Geometry: see drawing. Coordinates: mm, zero at the bounding-box minimum. Coordinates: 2 decimals unless noted, no trailing zeros. Loops run counter-clockwise (first coordinate to the right, second up) from the corner with the lowest first, then second, coordinate; pieces in that order, holes last. Notation, with made-up numbers: (20.5, 85.25) - (41.5, 85.25) arc R30 cw to (41.5, 123.25) - close; hole circle Ø8 at (19.5, -39.5). An arc over 180 degrees is marked (long way). Write item = value, one per line. Start each with the question number.
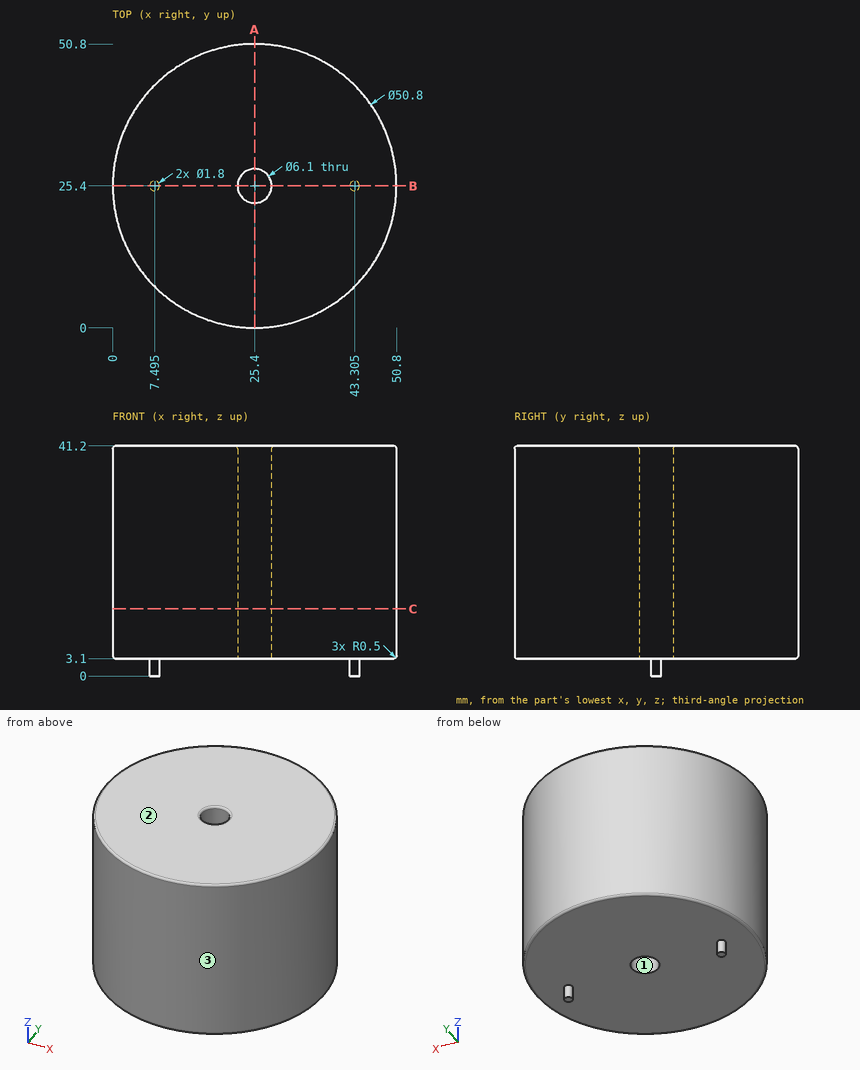
Item 1: Draft query along Y for the marked faces 1, 2 and 3. Return one class per face: released by +Y, released by -Y, zero draft, split by the parting line, or undercut.
Item 2: First-contact query: pin 1 (8 mm diameter, centred on x = 17, z = 4.5, fed in from -Y); pin 2 (2 mm diameter, centred on x = 24, z = 10.5, fed in from -Y); pin 3 (5 mm diameter, centred on x = 34.5, z = 9.5, fed in from -Y); pin 4 (5.5 mm diameter, centred on x = 25.4, y = 25.4, fed in from -Z). Flat tips, straight axial feed; report the tip coordinate or a pass-through.
Item 3: Cut plane C-C (z = 12). Return the cut outline in (x, y), then the cut area to 3 significant figures.
Item 4: Cut plane B-B (y = 25.4). Return the cut outline in (x, z) (3 decimals), then the cut area to 3 significant figures.
Item 5: Cut plane A-A (x = 25.4). Return the cut outline in (y, z).
Item 6: Material intervals for L1, parallel to Y at x = 25.4, z = 22; L2, parallel to Z at x = 12, y = 16.5; L3, parallel to X at y = 25, z = 26, sorted ascending. Write a range as [from, to].
Responses:
q1.face_1 = undercut
q1.face_2 = zero draft
q1.face_3 = split by the parting line
q2.pin_1 = 0.38
q2.pin_2 = 0
q2.pin_3 = 0.87
q2.pin_4 = through
q3.outline = circle Ø50.8 at (25.4, 25.4); hole circle Ø6.1 at (25.4, 25.4)
q3.area = 2,000 mm2
q4.outline = (0, 3.6) arc R0.5 ccw to (0.5, 3.1) - (6.595, 3.1) - (6.595, 0) - (8.395, 0) - (8.395, 3.1) - (22.35, 3.1) - (22.35, 40.7) arc R0.5 ccw to (21.85, 41.2) - (0.5, 41.2) arc R0.5 ccw to (0, 40.7) - close; (28.45, 3.1) - (42.405, 3.1) - (42.405, 0) - (44.205, 0) - (44.205, 3.1) - (50.3, 3.1) arc R0.5 ccw to (50.8, 3.6) - (50.8, 40.7) arc R0.5 ccw to (50.3, 41.2) - (28.95, 41.2) arc R0.5 ccw to (28.45, 40.7) - close
q4.area = 1,710 mm2
q5.outline = (0, 3.6) arc R0.5 ccw to (0.5, 3.1) - (22.35, 3.1) - (22.35, 40.7) arc R0.5 ccw to (21.85, 41.2) - (0.5, 41.2) arc R0.5 ccw to (0, 40.7) - close; (28.45, 3.1) - (50.3, 3.1) arc R0.5 ccw to (50.8, 3.6) - (50.8, 40.7) arc R0.5 ccw to (50.3, 41.2) - (28.95, 41.2) arc R0.5 ccw to (28.45, 40.7) - close
q6.L1 = [0, 22.35], [28.45, 50.8]
q6.L2 = [3.1, 41.2]
q6.L3 = [0, 22.38], [28.42, 50.8]
